For this review, take the finished solid that the model builds, in its own axes (mm). A direction names the side the tool comes from. Give positions to 0.01 mm unless a question says otherwise; leave off trailing zeros. Loops run counter-clockwise (first coordinate to the right, second up) from the corner with the lowest first, then second, coordinate; pieces in that order, holes last.
```python
from build123d import *

# Parameters (mm, degrees)
F0_W     = 122.814625
F0_H     = 30.703664
F1_DEPTH = 76.2
F2_T     = -2.54


with BuildPart() as f1:
    # F0 (on Front) → F1 (new body)
    with BuildSketch(Plane.XZ):
        with Locations((-32.36334, 38.172156)):
            Rectangle(F0_W, F0_H)
    extrude(amount=F1_DEPTH)

    # F2
    f2_openings = [f1.faces().sort_by_distance(p)[0] for p in [
        (-32.36334, -38.1, 53.523988),
    ]]
    offset(amount=F2_T, openings=f2_openings)


solid = f1.part
```
Q1. Machinability: for faces 1 (the flat face through (26.504, -38, 39)), 2 (the flat face through (-33, -38, 22.82)), which of the approach directions +Z, -Z, +X, -X, +Y, -Y give a long, thin tool a straight path to every point of the face, cutting with its end or side? Answer none if there is none.
Answers:
face 1: +Z
face 2: -Z, +X, -X, +Y, -Y
Q2. Consider section B-B on z = 33. Give the boundary of the cut face in (x, y), plus the area to 3 significant figures.
Answers:
outline: (-93.77, -76.2) - (29.04, -76.2) - (29.04, 0) - (-93.77, 0) - close; hole (-91.23, -73.66) - (26.5, -73.66) - (26.5, -2.54) - (-91.23, -2.54) - close
area: 985 mm2
Q3. Mouldability with a two-part tool opening along Y and no side actions: class faces 3 (the flat face through (-33, -2.54, 40)), 4 (the flat face through (-33, 0, 38)), 5 (the flat face through (-93.771, -38, 38)) as +Y half, -Y half, draft (parallel to the pull), parting line (faces both ways), or undercut.
Answers:
face 3: undercut
face 4: +Y half
face 5: draft
Q4. For probe 1 along X at (y, z) = (-7, 35); probe 2 along Y at (x, z) = (6.5, 42); probe 3 along Z at (x, y) = (-86.5, -49), list the stretches that pass through material, from the lowest coordinate up.
Answers:
probe 1: x = -93.77 to -91.23, 26.5 to 29.04
probe 2: y = -76.2 to -73.66, -2.54 to 0
probe 3: z = 22.82 to 25.36
Q5. Consider section C-C on x = -63. Give the boundary of the cut face in (y, z), plus the area to 3 significant figures.
Answers:
outline: (-76.2, 22.82) - (0, 22.82) - (0, 53.52) - (-2.54, 53.52) - (-2.54, 25.36) - (-73.66, 25.36) - (-73.66, 53.52) - (-76.2, 53.52) - close
area: 337 mm2
Q6. Consider section A-A on y = -31. Give the boundary of the cut face in (x, z), plus the area to 3 significant figures.
Answers:
outline: (-93.77, 22.82) - (29.04, 22.82) - (29.04, 53.52) - (26.5, 53.52) - (26.5, 25.36) - (-91.23, 25.36) - (-91.23, 53.52) - (-93.77, 53.52) - close
area: 455 mm2
Q7. For pin 1 Ø4 at (x, y) = (-25.5, -13.5) entering from +Z, flat-tipped, find the tip position at first contact; note if it passes through.
Answers:
pin 1: stops at z = 25.36
